Design review of the part built by this model. Coordinates are the model's own, in mm. A direction names the side the tool comes from. Coordinates: 2 decimals unless noted, no trailing zeros. Write each loop counter-clockwise with the first axis right and the second up, starting at its lowest first coordinate (ties: lowest second). Pieces come first, ordered by that corner, then holes. Notation, with made-up numbers: M 35.5,-13 L 66.5,-13 A22 ccw 66.5,-6 Z; hole C -33.5,4 d2. An arc over 180 degrees is marked long. Write each question's results on one line, items separated by ' | '. Start each with the question number.
Autodesk Inventor part; units mm, degrees
ref_plane "YZ Plane" through (0, 0, 0) normal (1, 0, 0) x (0, 1, 0)
ref_plane "XZ Plane" through (0, 0, 0) normal (0, 1, 0) x (-1, 0, 0)
ref_plane "XY Plane" through (0, 0, 0) normal (0, 0, 1) x (1, 0, 0)
sketch "Esboço1" plane through (0, 0, 0) normal (0, 1, 0) x (-1, 0, 0)
  circle A0 centre (0, 0) radius 1.25
  arc A1 (-2.0603, -3.4286) -> (-2.0603, 3.4286) centre (0, 0) ccw
  circle A2 centre (-25, 0) radius 1.25
  arc A3 (-22.9397, 3.4286) -> (-22.9397, -3.4286) centre (-25, 0) ccw
  line L0 (-3.6056, -3) -> (-21.3944, -3)
  line L1 (-3.6056, 3) -> (-21.3944, 3)
  arc A4 (-2.0603, -3.4286) -> (-3.6056, -3) centre (-3.6056, -6) ccw
  arc A5 (-3.6056, 3) -> (-2.0603, 3.4286) centre (-3.6056, 6) ccw
  arc A6 (-21.3944, -3) -> (-22.9397, -3.4286) centre (-21.3944, -6) ccw
  arc A7 (-22.9397, 3.4286) -> (-21.3944, 3) centre (-21.3944, 6) ccw
  point P0 (-2.6458, -3)
  point P1 (-22.3542, -3)
  point P2 (-2.6458, 3)
  point P3 (-22.3542, 3)
  dimension "d1" = 2.5
  dimension "d3" = 6
  dimension "d5" = 3
  dimension "d6" = 25
  dimension "d10" = 4
extrude "Extrusão1" add sketch "Esboço1" along normal blind 2.5
fillet "Arredondamento1" radius 0.3 16 edges at (22.1962, 0, 3.1091) (29, 0, 0) (22.1962, 0, -3.1091) (12.5, 0, -3) (2.8038, 0, -3.1091) (-4, 0, 0) (2.8038, 0, 3.1091) (12.5, 0, 3) (22.1962, 2.5, 3.1091) (29, 2.5, 0) (22.1962, 2.5, -3.1091) (12.5, 2.5, -3) (2.8038, 2.5, -3.1091) (-4, 2.5, 0) (2.8038, 2.5, 3.1091) (12.5, 2.5, 3)
sketch "Esboço2" plane through (0, 2.5, 0) normal (0, 1, 0) x (1, 0, 0)
  circle A0 centre (0, 0) radius 2.5
  circle A1 centre (25, 0) radius 1.25
  circle A2 centre (25, 0) radius 2.5
  dimension "d11" = 5
extrude "Extrusão2" cut sketch "Esboço2" against normal blind 1.5
properties part number "_3DPrint"
Item 1: For faces 3 (the cylindrical face through (2.793, 1.237, 3.112)), 4 (the flat face through (1, 1, -1)), 5 (the cylindrical face through (22.207, 1.237, -3.112)), list the 3-axis set-ups (+Z, -Z, +X, -X, +Y, -Y) from which the entire face can be reached by the end or side of a thin tool; tool diameter is ignored.
Item 2: Wall thickness on L1, parallel to X at y = 1.45, z = 0; L2, parallel to Z at x = 0, y = 0.55; L3, parallel to X at y = 1.8, z = -1.5: over which ranges is each line inside the solid? List them lowest first.
Item 3: We need section B-B on y = 1.4. State the section outline as (x, z) points.
Item 4: We need section A-A on x = 25. State the section outline as (y, z) points, then the cut area to 3 significant figures.
Item 5: Draft analysis for pull direction X (two halves, no side actions). For faces 1 (the cylindrical face through (-0.54, 1.76, 2.44)), 2 (the flat face through (13, 2.5, 0)), state which applies: released by +X, released by -X, zero draft, split by the parting line, or undercut.
Item 6: Insertion check: pin 1 Ø1.5 at (y, z) = (1.5, -1.5) entering from +X; pin 2 Ø1.5 at (y, z) = (1.5, -2) entering from -X; pin 3 Ø1.5 at (x, z) = (24.5, 1) entering from +Y. Each pin has a flat end and moves straight along its axis. Give the tip position at first contact, or say it passes through.
Item 7: We need section D-D on x = 11. State the section outline as (y, z) points.
Item 8: We need section C-C on z = 0. State the section outline as (x, y) points.
Answer:
1) face 3: +Z, +Y, -Y | face 4: +Y | face 5: -Z, +Y, -Y
2) L1: x = -4 to -2.5, 2.5 to 22.5, 27.5 to 29 | L2: z = -4 to -1.25, 1.25 to 4 | L3: x = -3.71 to -2, 2 to 23, 27 to 28.71
3) outline: M 2.06,-3.43 A3 cw 3.61,-3 L 21.39,-3 A3 cw 22.94,-3.43 A4 ccw long 22.94,3.43 A3 cw 21.39,3 L 3.61,3 A3 cw 2.06,3.43 A4 ccw long Z; hole C 0,0 d5; hole C 25,0 d5
4) outline: M 0,-3.7 A0.3 ccw 0.3,-4 L 2.2,-4 A0.3 ccw 2.5,-3.7 L 2.5,-2.5 L 1,-2.5 L 1,-1.25 L 0,-1.25 Z; M 0,1.25 L 1,1.25 L 1,2.5 L 2.5,2.5 L 2.5,3.7 A0.3 ccw 2.2,4 L 0.3,4 A0.3 ccw 0,3.7 Z | area: 9.92 mm^2
5) face 1: undercut | face 2: zero draft
6) pin 1: stops at x = 28.93 | pin 2: stops at x = -3.8 | pin 3: stops at y = 1
7) outline: M 0,-2.7 A0.3 ccw 0.3,-3 L 2.2,-3 A0.3 ccw 2.5,-2.7 L 2.5,2.7 A0.3 ccw 2.2,3 L 0.3,3 A0.3 ccw 0,2.7 Z
8) outline: M -4,0.3 A0.3 ccw -3.7,0 L -1.25,0 L -1.25,1 L -2.5,1 L -2.5,2.5 L -3.7,2.5 A0.3 ccw -4,2.2 Z; M 1.25,0 L 23.75,0 L 23.75,1 L 22.5,1 L 22.5,2.5 L 2.5,2.5 L 2.5,1 L 1.25,1 Z; M 26.25,0 L 28.7,0 A0.3 ccw 29,0.3 L 29,2.2 A0.3 ccw 28.7,2.5 L 27.5,2.5 L 27.5,1 L 26.25,1 Z
